from build123d import *

# Parameters (mm, degrees)
FILLET1_R = 0.127


with BuildPart() as part:
    # Sketch2 → Revolve1 (revolve)
    with BuildSketch(Plane.XY):
        with BuildLine():
            Line((-6.35, 0), (-6.35, 6.746875))
            ThreePointArc((-6.35, 6.746875), (-6.001274011, 7.588774011), (-5.159375, 7.9375))
            Line((-5.159375, 7.9375), (-3.175, 7.9375))
            Line((-3.175, 7.9375), (-3.175, 3.175))
            Line((-3.175, 3.175), (-1.984375, 3.175))
            Line((-1.984375, 3.175), (-1.984375, 0))
            Line((-1.984375, 0), (-6.35, 0))
        make_face()
    revolve(axis=Axis((0, 0, 0), (0, 1, 0)))

    # Fillet1
    fillet1_edges = [part.edges().sort_by_distance(p)[0] for p in [
        (3.175, 7.9375, 0),
    ]]
    fillet(fillet1_edges, radius=FILLET1_R)


solid = part.part
Part model, mm, in its own coordinate system. A direction names the side the tool comes from. Give positions to 0.01 mm unless a question says otherwise; leave off trailing zeros. Loops run counter-clockwise (first coordinate to the right, second up) from the corner with the lowest first, then second, coordinate; pieces in that order, holes last. Notation, with made-up numbers: M 23,72 L 80,72 A25 ccw 80,84 Z; hole C -26,75.25 d7. An arc over 180 degrees is marked long. Put each result on its own line as item: value. Start each with the question number.
1) 3-axis set-ups, long thin cutter, end or side, ignore diameter. For faces 1 (the flat face through (1, 0, 2)), 2 (the cylindrical face through (0.69, 5.46, -3.1)): which of +Z, -Z, +X, -X, +Y, -Y reach the whole face in a straight line?
2) Pull direction Z, two halves, no side cores. Call faces 3 (the cylindrical face through (0.43, 1.565, -1.937)), 4 (the flat face through (-1.1, 7.938, -3.4)), 5 (the cylindrical face through (1.38, 3.42, -6.2)): +Z half, -Z half, draft (parallel to the pull), parting line (faces both ways), or undercut.
3) Flat gauge pins, fed straight in: pin 1 (4 mm diameter, centred on y = 5, z = -4.5, fed in from -X); pin 2 (3 mm diameter, centred on y = 2, z = -1.5, fed in from -X); pin 3 (3 mm diameter, centred on x = -2.5, y = 7, fed in from +Z); pin 4 (5 mm diameter, centred on x = 0, z = 0, fed in from +Y) (3 decimals). Where does each tip first touch, or does it go through?
4) Probe probe 1 along Z at (x, y) = (0, 5.45) (3 decimals); probe 2 along Z at (x, y) = (5.5, 3); probe 3 along Z at (x, y) = (-1, 4.25). List the from-to ranges inside material, lowest first.
5) Saw through at C-C (y = 3). List the corners of the cut face in (x, z), then the cut area to 3 significant figures.
6) Saw through at D-D (y = 6.5). List the corners of the cut face in (x, z) (3 decimals), then the cut area to 3 significant figures.
Numbers:
1. face 1: +Z, -Z, +X, -X, -Y
1. face 2: +Y
2. face 3: undercut
2. face 4: draft
2. face 5: parting line
3. pin 1: x = -5.84
3. pin 2: x = -6.35
3. pin 3: z = 6.27
3. pin 4: y = 3.175
4. probe 1: -6.35 to -3.175, 3.175 to 6.35
4. probe 2: -3.17 to 3.17
4. probe 3: -6.27 to -3.01, 3.01 to 6.27
5. outline: C 0,0 d12.7; hole C 0,0 d3.97
5. area: 114 mm^2
6. outline: C 0,0 d12.7; hole C 0,0 d6.35
6. area: 95.0 mm^2
